Build history of the part. All positions in model axes, mm. Face numbers are marked on the shaded views. Coordinates: 2 decimals unless noted, no trailing zeros. Loops run counter-clockwise (first coordinate to the right, second up) from the corner with the lowest first, then second, coordinate; pieces in that order, holes last.
Item 1: Cut at A-A (z = 19.5). List the corners of the cut face in (x, y), and give its area (3 significant figures).
Item 2: Cut at B-B (y = 0). List the corners of the cut face in (x, z), and give its area (3 significant figures).
Item 3: Mould opens along Y. For the marked faces 1, 2, 3 and 4 say: released by +Y, released by -Y, zero draft, split by the parting line, or undercut.
Item 4: Drill centre lines: line 1 along Y through (x, z) = (0, 10.5); line 2 along Y through (x, z) = (-5.5, 11.5); line 3 along X through (y, z) = (-16, 32.5). Where is each one in solid material? Low to high.
Item 5: Cut at C-C (x = 0). List the corners of the cut face in (y, z).
Item 6: Flat gauge pins, fed straight in: pin 1 (10 mm diameter, centred on x = 29, z = 13, fed in from +Y); pin 2 (5 mm diameter, centred on x = 24, z = 26, fed in from +Y); pin 3 (5 mm diameter, centred on x = -30.5, y = 5.5, fed in from -Z); pin 4 (3 mm diameter, centred on x = -23, y = 28.5, fed in from +Z). Where does each tip first touch, or does it go through?
from build123d import *

# Parameters (mm, degrees)
F0_R     = 20.25
F1_DEPTH = 36
F2_SIZE  = 2


with BuildPart() as f1:
    # F0 (on Top) → F1 (new body)
    with BuildSketch(Plane.XY):
        Polygon((21.8537385337, -33.9962857594), (40.3685163688, 1.9277498582), (18.5147778351, 35.9240356175), (-21.8537385337, 33.9962857594), (-40.3685163688, -1.9277498582), (-18.5147778351, -35.9240356175), align=None)
        Circle(F0_R, mode=Mode.SUBTRACT)
    extrude(amount=F1_DEPTH)

    # F2
    f2_edges = [f1.edges().sort_by_distance(p)[0] for p in [
        (-20.25, 0, 36),
        (-20.25, 0, 0),
    ]]
    chamfer(f2_edges, length=F2_SIZE)

    # F5 (on 3pt) → F6 (revolve, cut)
    with BuildSketch(Plane(origin=(0, 0, 0), x_dir=(0.998861734, 0.0476994386, 0), z_dir=(0.0476994386, -0.998861734, 0))):
        Polygon((35, 37.1090732515), (35, 36), (44.6592582629, 33.411809549), (44.6592582629, 39.6752795403), align=None)
        Polygon((35, -1.1090732515), (44.6592582629, -3.6752795403), (44.6592582629, 2.588190451), (35, 0), align=None)
    revolve(axis=Axis((0, 0, 0), (0, 0, -1)), mode=Mode.SUBTRACT)


solid = f1.part
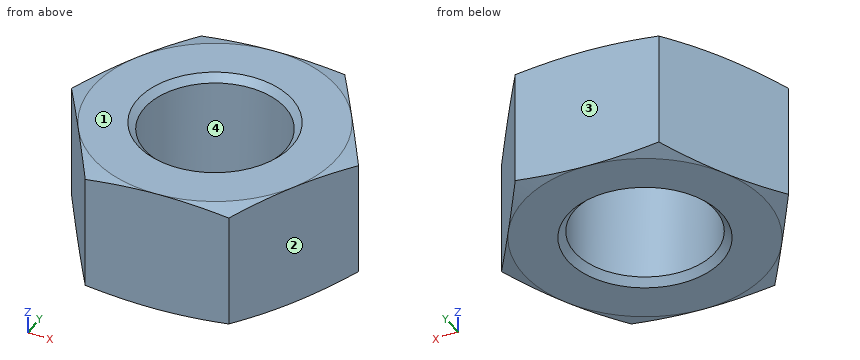
Filled sheet:
1. outline: (-40.37, -1.93) - (-18.51, -35.92) - (21.85, -34) - (40.37, 1.93) - (18.51, 35.92) - (-21.85, 34) - close; hole circle Ø40.5 at (0, 0)
1. area: 2,960 mm2
2. outline: (-39.37, 1.17) - (-35, 0) - (-22.25, 0) - (-20.25, 2) - (-20.25, 34) - (-22.25, 36) - (-35, 36) - (-39.37, 34.83) - close; (20.25, 2) - (22.25, 0) - (35, 0) - (39.37, 1.17) - (39.37, 34.83) - (35, 36) - (22.25, 36) - (20.25, 34) - close
2. area: 1,360 mm2
3. face 1: zero draft
3. face 2: released by -Y
3. face 3: released by +Y
3. face 4: undercut
4. line 1: y = -35.04 to -20.25, 20.25 to 35.04
4. line 2: y = -35.3 to -19.49, 19.49 to 34.78
4. line 3: x = -31.32 to -12.41, 12.41 to 31.13
5. outline: (-35.04, 0.01) - (-35, 0) - (-22.25, 0) - (-20.25, 2) - (-20.25, 34) - (-22.25, 36) - (-35, 36) - (-35.04, 35.99) - close; (20.25, 2) - (22.25, 0) - (35, 0) - (35.04, 0.01) - (35.04, 35.99) - (35, 36) - (22.25, 36) - (20.25, 34) - close
6. pin 1: stops at y = 27.39
6. pin 2: stops at y = 31.28
6. pin 3: stops at z = 0
6. pin 4: stops at z = 35.97
